```python
from build123d import *

# Parameters (mm, degrees)
F0_R     = 3
F1_DEPTH = 10
F3_DEPTH = 40
F5_DEPTH = 25
F6_R     = 3
F6_R_2   = 2
F7_DEPTH = 15
F8_R     = 1.9959654756
F9_DEPTH = 19.5


with BuildPart() as f1:
    # F0 (on Top) → F1 (new body)
    with BuildSketch(Plane.XY):
        with BuildLine():
            Line((0, -6), (16.3284806108, -33.7584170384))
            ThreePointArc((16.3284806108, -33.7584170384), (0, 37.5), (-16.3284806108, -33.7584170384))
            Line((-16.3284806108, -33.7584170384), (0, -6))
        make_face()
        Circle(F0_R, mode=Mode.SUBTRACT)
    extrude(amount=F1_DEPTH)

    # F2 (on face) → F3 (join)
    with BuildSketch(Plane.XY.offset(10)):
        with BuildLine():
            Line((-2.2077877193, -9.7532391228), (-7.4003026682, -18.5805145359))
            ThreePointArc((-7.4003026682, -18.5805145359), (0, -20), (7.4003026682, -18.5805145359))
            Line((7.4003026682, -18.5805145359), (2.2077877193, -9.7532391228))
            ThreePointArc((2.2077877193, -9.7532391228), (0, -10), (-2.2077877193, -9.7532391228))
        make_face()
        with BuildLine():
            ThreePointArc((7.4003026682, -18.5805145359), (16.5530367813, -11.2248373404), (20, 0))
            ThreePointArc((20, 0), (-11.2248373404, 16.5530367813), (-7.4003026682, -18.5805145359))
            Line((-7.4003026682, -18.5805145359), (-2.2077877193, -9.7532391228))
            ThreePointArc((-2.2077877193, -9.7532391228), (-6.2418796371, 7.8127420664), (10, 0))
            ThreePointArc((10, 0), (7.8127420664, -6.2418796371), (2.2077877193, -9.7532391228))
            Line((2.2077877193, -9.7532391228), (7.4003026682, -18.5805145359))
        make_face()
    extrude(amount=F3_DEPTH)

    # F4 (on face) → F5 (cut)
    with BuildSketch(Plane.XY.offset(50)):
        with BuildLine():
            ThreePointArc((-1, -19.9749843554), (0, -20), (1, -19.9749843554))
            Line((1, -19.9749843554), (1, -9.9498743711))
            ThreePointArc((1, -9.9498743711), (0, -10), (-1, -9.9498743711))
            Line((-1, -9.9498743711), (-1, -19.9749843554))
        make_face()
    extrude(amount=-F5_DEPTH, mode=Mode.SUBTRACT)

    # F6 (on face) → F7 (join)
    with BuildSketch(Plane.XY.offset(10)):
        Circle(F6_R)
        Circle(F6_R_2, mode=Mode.SUBTRACT)
    extrude(amount=-F7_DEPTH)

    # F8 (on Right) → F9 (cut, symmetric)
    with BuildSketch(Plane.YZ):
        with Locations((-14.9785717949, 41.0785749555)):
            Circle(F8_R)
    extrude(amount=F9_DEPTH, both=True, mode=Mode.SUBTRACT)


solid = f1.part
```
Geometry check sheet. Reference: the model listing, model coordinates, mm. A direction names the side the tool comes from. Coordinates: 2 decimals unless noted, no trailing zeros. Order: outer loops, then holes, each group sorted by start corner. A loop starts at its lowest first (then second) coordinate and runs counter-clockwise, first axis right, second up. Notation, with made-up numbers: (-11, 41) - (-1, 41) arc R21 ccw to (-1, 49) - close; hole circle Ø2 at (47.25, 1). An arc over 180 degrees is marked (long way). Use one line per item in the form item = value.
1. Scan lines: line 1 (Z direction, x = 2, y = 20); line 2 (Z direction, x = -10.5, y = -0.5); line 3 (Y direction, x = -2, z = 42). Record each from-to range of solid material in increasing order.
Here are the results:
line_1 = 0 to 10
line_2 = 0 to 50
line_3 = -19.9 to -16.75, -13.21 to -9.8, 9.8 to 19.9
2. Section check A-A (z = 33). Record the boundary of the cut face in (x, y), then the cut area to 3 significant figures.
Here are the results:
outline = (-1, -19.97) - (-1, -9.95) arc R10 cw (long way) to (1, -9.95) - (1, -19.97) arc R20 ccw (long way) to start
area = 922 mm²
3. Access from +Z, -Z, +X, -X, +Y, -Y to the whole of each face (thin tool, end or side, straight path). Record for faces 5 (the face through (1, -15, 38)), 6 (the face through (-8.279, -20.074, 4.93)), 7 (the face through (-8.9, 18.2, 10)).
Here are the results:
face_5 = +Z, -Y
face_6 = -Z, -Y
face_7 = +Z
4. Gauge pin test, flat ends, axial feed: pin 1 (2 mm diameter, centred on x = 26.5, y = -11.5, fed in from -Z); pin 2 (6 mm diameter, centred on x = -1.5, y = 4.5, fed in from +Z); pin 3 (6.5 mm diameter, centred on y = -14.98, z = 41.08, fed in from -X); pin 4 (3.5 mm diameter, centred on x = 0, y = 0, fed in from -Z). Record the tip position at first contact, or that the pin passes through.
Here are the results:
pin_1 = 0
pin_2 = 10
pin_3 = -16.2
pin_4 = through
5. Section check C-C (y = 18.5). Record the boundary of the cut face in (x, z), then the cut area to 3 significant figures.
Here are the results:
outline = (-32.62, 0) - (32.62, 0) - (32.62, 10) - (7.6, 10) - (7.6, 50) - (-7.6, 50) - (-7.6, 10) - (-32.62, 10) - close
area = 1,260 mm²
6. Section check D-D (x = -9). Record the boundary of the cut face in (y, z), then the cut area to 3 significant figures.
Here are the results:
outline = (-21.3, 0) - (36.4, 0) - (36.4, 10) - (17.86, 10) - (17.86, 50) - (4.36, 50) - (4.36, 10) - (-4.36, 10) - (-4.36, 50) - (-17.86, 50) - (-17.86, 10) - (-21.3, 10) - close; hole circle Ø3.99 at (-14.98, 41.08)
area = 1,640 mm²
7. Section check B-B (y = -25.5). Record the boundary of the cut face in (x, z), then the cut area to 3 significant figures.
Here are the results:
outline = (-27.5, 0) - (-11.47, 0) - (-11.47, 10) - (-27.5, 10) - close; (11.47, 0) - (27.5, 0) - (27.5, 10) - (11.47, 10) - close
area = 320 mm²
8. Draft check along X on faces 1 (the face through (-1, -15, 38)), 2 (the face through (-3, 0, -2)), 3 (the face through (-1, 10, 0)), 4 (the face through (8.05, -19.685, 4.93)). Enter one of: pulls with the +X half, pulls with the -X half, needs draft (parallel to the pull), parting line crosses it, or undercut.
Here are the results:
face_1 = undercut
face_2 = parting line crosses it
face_3 = needs draft
face_4 = undercut
